Could you check a few things on this model? Use its own coordinates, in mm. Face numbers are marked on the shaded views. A direction names the side the tool comes from. Give positions to 0.01 mm unless a question says otherwise; leave off trailing zeros. Order: outer loops, then holes, each group sorted by start corner. A loop starts at its lowest first (then second) coordinate and runs counter-clockwise, first axis right, second up. Notation, with made-up numbers: (9.25, 64) - (51.25, 64) arc R10 cw to (51.25, 73) - close; hole circle Ø11 at (38.5, -39.5). An arc over 180 degrees is marked (long way). Put each result on its own line as item: value.
from build123d import *

# Parameters (mm, degrees)
REVOLUTION001_ANGLE = -90
PAD008_DEPTH        = 1.75


with BuildPart() as m3din7991slot001:
    # Clone2D → Revolution001 (revolve)
    with BuildSketch(Plane.XY.offset(1.75)):
        Polygon((0, 0), (3, 0), (1.7, -1.3), (1.7, -40), (0, -40), align=None)
    revolve(axis=Axis((0, 0, 1.75), (0, 1, 0)), revolution_arc=REVOLUTION001_ANGLE)


with BuildPart() as slotquarter:
    # Sketch016 → Pad008 (new body)
    with BuildSketch(Plane.XY):
        Polygon((0, 0), (3, 0), (1.7, -1.3), (1.7, -40), (0, -40), align=None)
    extrude(amount=PAD008_DEPTH)

    # Fusion001: union M3DIN7991Slot001
    add(m3din7991slot001.part)


with BuildPart() as part_mirroring002:
    # Part__Mirroring002: instance of SlotQuarter
    add(slotquarter.part.mirror(Plane(origin=(0, 0, 0), x_dir=(0, -1, 0), z_dir=(1, 0, 0))))


with BuildPart() as fusion002:
    # Fusion002 base: copy of SlotQuarter
    add(slotquarter.part)

    # Fusion002: union Part__Mirroring002
    add(part_mirroring002.part)


with BuildPart() as part_mirroring003:
    # Part__Mirroring003: instance of Fusion002
    add(fusion002.part.mirror(Plane(origin=(0, 0, 0), x_dir=(0, 1, 0), z_dir=(0, 0, 1))))


with BuildPart() as refine_m3din7991boltslot:
    # Fusion003 base: copy of Fusion002
    add(fusion002.part)

    # Fusion003: union Part__Mirroring003
    add(part_mirroring003.part)


solid = refine_m3din7991boltslot.part
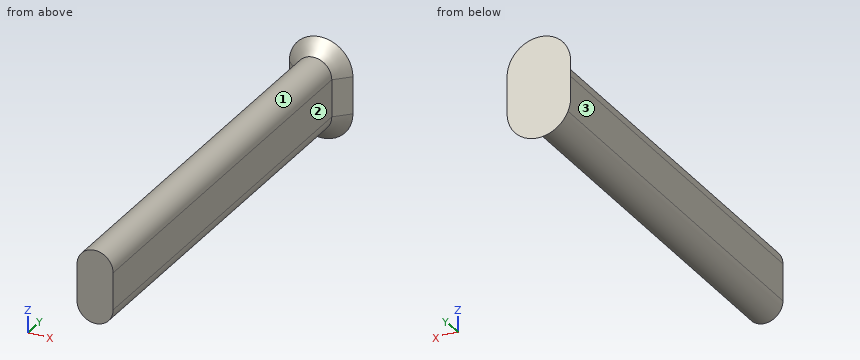
1) Suppose I cut it at A-A, the plane z = -0.5. List the corners of the cut face in (x, y) for me.
Filled in:
outline: (-3, 0) - (-1.7, -1.3) - (-1.7, -40) - (1.7, -40) - (1.7, -1.3) - (3, 0) - close
2) If I drill on line 1 (X direction, y = -9, z = -0.25); line 2 (Z direction, x = 0.6, y = -10); line 3 (Y direction, x = 2.3, z = 0.25), over which ranges is the centre line in solid material (lowest first)? Write a range as [from, to].
Filled in:
line 1: x = [-1.7, 1.7]
line 2: z = [-3.34, 3.34]
line 3: y = [-0.7, 0]
3) Suppose I cut it at B-B, the plane x = 0. List the corners of the cut face in (y, z) for me.
Filled in:
outline: (-40, -3.45) - (-1.3, -3.45) - (0, -4.75) - (0, 4.75) - (-1.3, 3.45) - (-40, 3.45) - close
4) I'm going to push flat-ended pins straight in: pin 1 (2 mm diameter, centred on x = 1.5, y = -19.5, fed in from -Z); pin 2 (5 mm diameter, centred on y = -18.5, z = -0.5, fed in from -X); pin 3 (3 mm diameter, centred on y = -13, z = 0, fed in from +X). Where does each tip first touch, or does it pass through?
Filled in:
pin 1: stops at z = -3.37
pin 2: stops at x = -1.7
pin 3: stops at x = 1.7
5) Suppose I cut it at C-C, the plane y = -25.5. List the corners of the cut face in (x, z) for me, and give its area (3 significant figures).
Filled in:
outline: (-1.7, -1.75) arc R1.7 ccw to (1.7, -1.75) - (1.7, 1.75) arc R1.7 ccw to (-1.7, 1.75) - close
area: 21.0 mm^2
6) Which directions (+Z, -Z, +X, -X, +Y, -Y) give clear straight access to the entire face, cutting with the end or side of a thin tool? Please do the marked faces 1, 2 and 3.
Filled in:
face 1: +Z, -Y
face 2: +Z, -Z, +X, -Y
face 3: +Z, -Z, -X, -Y
